CAD build for the part. Positions are in the model's coordinates, mm. Give positions to 0.01 mm unless a question says otherwise; leave off trailing zeros. Write each loop counter-clockwise with the first axis right and the second up, starting at its lowest first coordinate (ties: lowest second). Pieces come first, ordered by that corner, then holes. Notation, with made-up numbers: (-18.75, 26) - (38.25, 26) arc R19 ccw to (38.25, 38) - close; hole circle Ø1 at (-16.75, 41). An arc over 180 degrees is marked (long way). Put each result on its own line as item: value. Start each with the question number.
1. Drop a flat-ended pin along its axis: pin 1 (6.5 mm diameter, centred on x = 24.26, y = 6.35, fed in from +Z). Give the stop position or say it passes through.
2. Cut at D-D on x = 19.5. List the corners of the cut face in (y, z).
3. Wall check: line 1 (X direction, y = 6.35, z = 3); line 2 (X direction, y = 7, z = 5.5); line 3 (X direction, y = 9, z = 6.35) (3 decimals). Give the ranges that are in metal, low to high.
4. Cut at B-B on z = 6.35. List the corners of the cut face in (x, y) (3 decimals).
5. Cut at C-C on y = 1.5. List the corners of the cut face in (x, z) (3 decimals).
6. Mould opens along Z. For faces 1 (the flat face through (28, 0, 6)), 2 (the flat face through (28, 1, 12.7)), 3 (the cylindrical face through (45.316, 6.439, 7.308)) say: +Z half, -Z half, draft (parallel to the pull), parting line (faces both ways), or undercut.
7. Cut at A-A on y = 6.35. List the corners of the cut face in (x, z) (3 decimals), and give its area (3 significant figures).
from build123d import *

# Parameters (mm, degrees)
BOSS_EXTRU_2_DEPTH      = 12.7
ESQUISSE3_R             = 2.5
ENL_V_MAT_EXTRU_1_DEPTH = 12.7


with BuildPart() as part:
    # Esquisse1 → Boss.-Extru.2 (new body)
    with BuildSketch(Plane.XY):
        with BuildLine():
            Line((0, 0), (27.625, 0))
            Line((27.625, 0), (27.625, 2))
            ThreePointArc((27.625, 2), (18.759364844, 6.35), (27.625, 10.7))
            Line((27.625, 10.7), (27.625, 12.7))
            Line((27.625, 12.7), (0, 12.7))
            Line((0, 12.7), (0, 0))
        make_face()
    boss_extru_2 = extrude(amount=BOSS_EXTRU_2_DEPTH)

    # Esquisse3 → Enlèv. mat.-Extru.1 (cut)
    with BuildSketch(Plane(origin=(0, 12.7, 0), x_dir=(1, 0, 0), z_dir=(0, 1, 0))):
        with Locations((7.625, -6.35)):
            Circle(ESQUISSE3_R)
    enl_v_mat_extru_1 = extrude(amount=-ENL_V_MAT_EXTRU_1_DEPTH, mode=Mode.SUBTRACT)

    # Symétrie1: Boss.-Extru.2, Enlèv. mat.-Extru.1 across plane
    add(boss_extru_2.mirror(Plane(origin=(27.625, 12.7, 12.7), x_dir=(0, 0, 1), z_dir=(-1, 0, 0))))
    add(enl_v_mat_extru_1.mirror(Plane(origin=(27.625, 12.7, 12.7), x_dir=(0, 0, 1), z_dir=(-1, 0, 0))), mode=Mode.SUBTRACT)


solid = part.part
Report:
1. pin 1: passes through
2. outline: (0, 0) - (3.59, 0) - (3.59, 12.7) - (0, 12.7) - close; (9.11, 0) - (12.7, 0) - (12.7, 12.7) - (9.11, 12.7) - close
3. line 1: x = 0 to 18.76, 36.49 to 55.25
3. line 2: x = 0 to 5.27, 9.98 to 18.8, 36.45 to 45.27, 49.98 to 55.25
3. line 3: x = 0 to 5.125, 10.125 to 19.44, 35.81 to 45.125, 50.125 to 55.25
4. outline: (0, 0) - (5.125, 0) - (5.125, 12.7) - (0, 12.7) - close; (10.125, 0) - (45.125, 0) - (45.125, 12.7) - (10.125, 12.7) - close; (50.125, 0) - (55.25, 0) - (55.25, 12.7) - (50.125, 12.7) - close; hole (27.625, 2) arc R5.5 ccw (long way) to (27.625, 10.7) arc R5.5 ccw (long way) to start
5. outline: (0, 0) - (21.666, 0) - (21.666, 12.7) - (0, 12.7) - close; (26.853, 0) - (28.397, 0) - (28.397, 12.7) - (26.853, 12.7) - close; (33.584, 0) - (55.25, 0) - (55.25, 12.7) - (33.584, 12.7) - close; hole circle Ø5 at (7.625, 6.35); hole circle Ø5 at (47.625, 6.35)
6. face 1: draft
6. face 2: +Z half
6. face 3: undercut
7. outline: (0, 0) - (18.759, 0) - (18.759, 12.7) - (0, 12.7) - close; (36.491, 0) - (55.25, 0) - (55.25, 12.7) - (36.491, 12.7) - close; hole circle Ø5 at (7.625, 6.35); hole circle Ø5 at (47.625, 6.35)
7. area: 437 mm²
